Answer from the drawing. Dimensions are ordinates in mm from the lowest x, y and z of the part. A direction names the side the tool comes from. Give positions to 0.01 mm unless a question says otherwise; leave off trailing zeros. Loops run counter-clockwise (first coordinate to the right, second up) from the corner with the lowest first, then second, coordinate; pieces in that order, holes last.
Item 1: Each of these flat-tipped pins is pushed along its axis until it touches: pin 1 Ø6.5 at (y, z) = (564.5, 8.5) entering from +X; pin 2 Ø1 at (y, z) = (640, 157.5) entering from +X; pin 3 Ø24 at (y, z) = (521.5, 12.5) entering from -X. Where does it stop, or does it pass through?
Item 2: A tool of negligible diameter and unlimited length cuts with its end or side. For the marked faces 1, 2 and 3, from which of +Z, -Z, +X, -X, +Y, -Y can it reach the whole face along a straight path? Write none if from no direction.
Item 3: Consider line 1 along Y through (x, z) = (343.5, 9); line 2 along Z through (x, y) = (173.5, 402.5); line 3 along X through (y, z) = (669, 120). Determine where each line is inside the solid, lowest interval first.
Item 4: Section D-D, the plane x = 222 is taken. Give the vertices of the cut face in (y, z), and give its area (3 significant figures).
Item 5: Section C-C, the plane y = 398.5 is taken. Give the vertices of the cut face in (x, z), and give its area (3 significant figures).
Item 6: Section B-B, the plane z = 58.5 is taken. Give the vertices of the cut face in (x, y), and give its area (3 significant figures).
Item 7: Section A-A, the plane x = 48.5 is taken. Give the vertices of the cut face in (y, z).
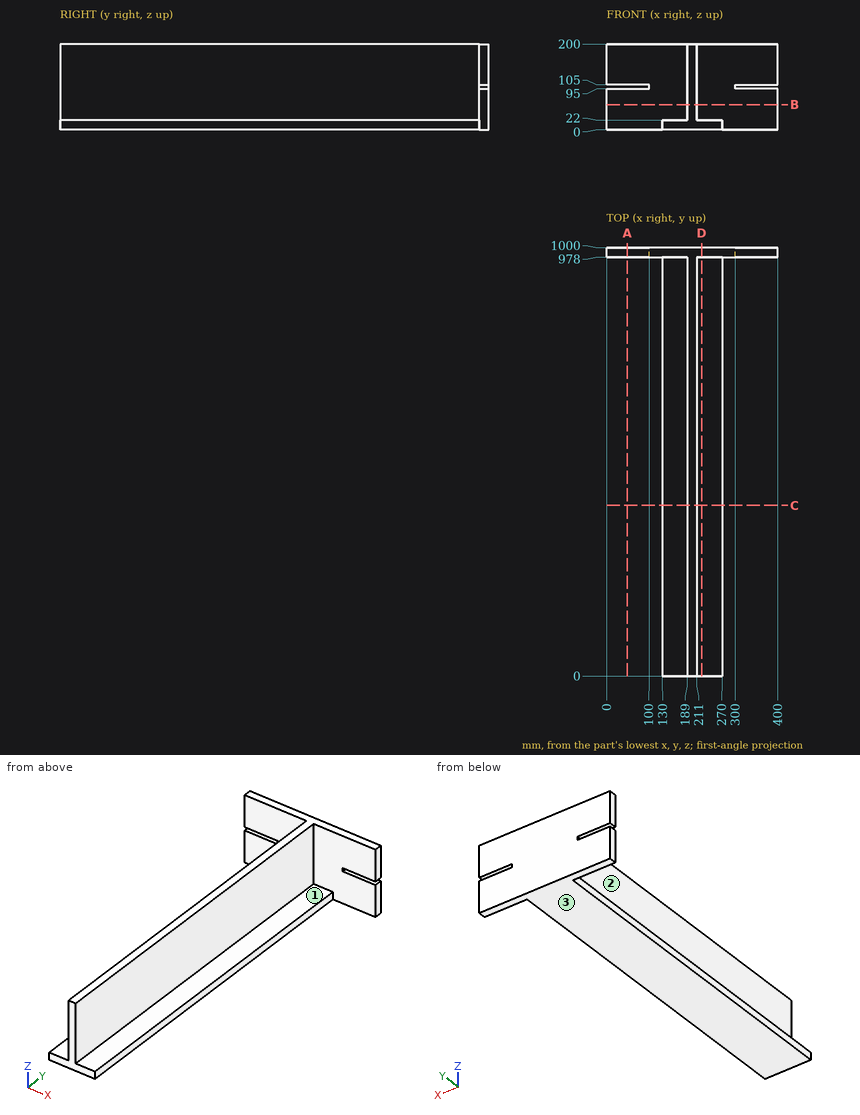
Worked answers:
1. pin 1: stops at x = 270
1. pin 2: stops at x = 211
1. pin 3: stops at x = 130
2. face 1: +Z, +X, -Y
2. face 2: +Z, -X, -Y
2. face 3: -Z, +X, -X, +Y, -Y
3. line 1: y = 978 to 1000
3. line 2: z = 0 to 22
3. line 3: x = 189 to 211
4. outline: (0, 0) - (1000, 0) - (1000, 200) - (978, 200) - (978, 22) - (0, 22) - close
4. area: 25,900 mm2
5. outline: (130, 0) - (270, 0) - (270, 22) - (211, 22) - (211, 200) - (189, 200) - (189, 22) - (130, 22) - close
5. area: 7,000 mm2
6. outline: (0, 978) - (189, 978) - (189, 0) - (211, 0) - (211, 978) - (400, 978) - (400, 1000) - (0, 1000) - close
6. area: 30,300 mm2
7. outline: (978, 0) - (1000, 0) - (1000, 95) - (978, 95) - close; (978, 105) - (1000, 105) - (1000, 200) - (978, 200) - close
